Here's how the part is built. I have some questions about the finished solid (model axes, mm). A direction names the side the tool comes from. Coordinates: 2 decimals unless noted, no trailing zeros. Order: outer loops, then holes, each group sorted by start corner. A loop starts at its lowest first (then second) coordinate and runs counter-clockwise, first axis right, second up. Notation, with made-up numbers: (-4.5, 35.5) -> (7.5, 35.5) arc R21 cw to (7.5, 50.5) -> close; hole circle Ø10 at (39.5, 89). An arc over 180 degrees is marked (long way). One line per item, written item: value. Start each with the question number.
```python
from build123d import *

# Parameters (mm, degrees)
EXTRUDE_BASE_DEPTH              = 2
SKETCH2_W                       = 57
SKETCH2_H                       = 68.2942
EXTRUDE_WALLS_DEPTH             = 25
SKETCH3_W                       = 8.390953786
SKETCH3_H                       = 13
CUT_USB_HOLE_DEPTH              = 75.121635616
SKETCH4_R                       = 1.375
CUT_CONNECTING_THRU_HOLES_DEPTH = 75.121635616
SKETCH5_R                       = 2.25
SKETCH5_R_2                     = 1.375
CUT_EXTRUDE3_DEPTH              = 0.5
SKETCH6_R                       = 1.125
CUT_CABLE_COVER_BOTTOM_DEPTH    = 75.121635616
SKETCH7_R                       = 1.125
CUT_CABLE_COVER_SIDE_DEPTH      = 2
SKETCH8_W                       = 3.5
SKETCH8_H                       = 10
EXTRUDE_HINGE_DEPTH             = 4
SKETCH9_R                       = 1.125
CUT_HINGE_HOLE_DEPTH            = 85.478484791
FILLET_HINGE_R                  = 1.75
SKETCH10_W                      = 40
SKETCH10_H                      = 5
CUT_NOTCH_DEPTH                 = 1.5
SKETCH11_W                      = 10
SKETCH11_H                      = 5
CUT_SIDE_NOTCH_DEPTH            = 1.5
FILLET_NOTCH_R                  = 1.5


with BuildPart() as part:
    # Sketch1 → Extrude Base (new body)
    with BuildSketch(Plane.XZ.offset(-16.914945084)):
        with BuildLine():
            Line((56.857940404, 38.199863775), (56.857940404, -32.594336225))
            ThreePointArc((56.857940404, -32.594336225), (56.198930662, -34.185326483), (54.607940404, -34.844336225))
            Line((54.607940404, -34.844336225), (-4.892059596, -34.844336225))
            ThreePointArc((-4.892059596, -34.844336225), (-6.483049854, -34.185326483), (-7.142059596, -32.594336225))
            Line((-7.142059596, -32.594336225), (-7.142059596, 38.199863775))
            ThreePointArc((-7.142059596, 38.199863775), (-6.483049854, 39.790854032), (-4.892059596, 40.449863775))
            Line((-4.892059596, 40.449863775), (54.607940404, 40.449863775))
            ThreePointArc((54.607940404, 40.449863775), (56.198930662, 39.790854032), (56.857940404, 38.199863775))
        make_face()
    extrude(amount=EXTRUDE_BASE_DEPTH)

    # Sketch2 → Extrude Walls (add)
    with BuildSketch(Plane.XZ.offset(-14.914945084)):
        with BuildLine():
            Line((56.857940404, -32.594336225), (56.857940404, 38.199863775))
            ThreePointArc((56.857940404, 38.199863775), (56.198930662, 39.790854032), (54.607940404, 40.449863775))
            Line((54.607940404, 40.449863775), (-4.892059596, 40.449863775))
            ThreePointArc((-4.892059596, 40.449863775), (-6.483049854, 39.790854032), (-7.142059596, 38.199863775))
            Line((-7.142059596, 38.199863775), (-7.142059596, -32.594336225))
            ThreePointArc((-7.142059596, -32.594336225), (-6.483049854, -34.185326483), (-4.892059596, -34.844336225))
            Line((-4.892059596, -34.844336225), (54.607940404, -34.844336225))
            ThreePointArc((54.607940404, -34.844336225), (56.198930662, -34.185326483), (56.857940404, -32.594336225))
        make_face()
        with Locations((24.857940404, 2.802763775)):
            Rectangle(SKETCH2_W, SKETCH2_H, mode=Mode.SUBTRACT)
    extrude(amount=EXTRUDE_WALLS_DEPTH)

    # Sketch3 → Cut USB Hole (cut, through all)
    with BuildSketch(Plane.XZ.offset(-14.914945084)):
        with Locations((0.553417297, 27.849863775)):
            Rectangle(SKETCH3_W, SKETCH3_H)
    extrude(amount=-CUT_USB_HOLE_DEPTH, mode=Mode.SUBTRACT)

    # Sketch4 → Cut Connecting Thru Holes (cut, through all)
    with BuildSketch(Plane.XZ.offset(-14.914945084)):
        with Locations((50.982940404, 34.574863775)):
            Circle(SKETCH4_R)
        with Locations((50.982940404, -28.969336225)):
            Circle(SKETCH4_R)
        with Locations((-1.267059596, -28.969336225)):
            Circle(SKETCH4_R)
        with Locations((50.982940404, 2.802763775)):
            Circle(SKETCH4_R)
        with Locations((7.12389419, 21.124863775)):
            Circle(SKETCH4_R)
    extrude(amount=-CUT_CONNECTING_THRU_HOLES_DEPTH, mode=Mode.SUBTRACT)

    # Sketch5 → Cut-Extrude3 (cut)
    # profile 1 of 5: a face of its own
    with BuildSketch(Plane.XZ.offset(-14.914945084)):
        with Locations((7.12389419, 21.124863775)):
            Circle(SKETCH5_R)
        with Locations((7.12389419, 21.124863775)):
            Circle(SKETCH5_R_2, mode=Mode.SUBTRACT)
    # profile 2 of 5: a face of its own
    with BuildSketch(Plane.XZ.offset(-14.914945084)):
        with Locations((50.982940404, 34.574863775)):
            Circle(SKETCH5_R)
    # profile 3 of 5: a face of its own
    with BuildSketch(Plane.XZ.offset(-14.914945084)):
        with Locations((50.982940404, 2.802763775)):
            Circle(SKETCH5_R)
    # profile 4 of 5: a face of its own
    with BuildSketch(Plane.XZ.offset(-14.914945084)):
        with Locations((50.982940404, -28.969336225)):
            Circle(SKETCH5_R)
    # profile 5 of 5: a face of its own
    with BuildSketch(Plane.XZ.offset(-14.914945084)):
        with Locations((-1.267059596, -28.969336225)):
            Circle(SKETCH5_R)
    extrude(amount=-CUT_EXTRUDE3_DEPTH, mode=Mode.SUBTRACT)

    # Sketch6 → Cut Cable Cover Bottom (cut, through all)
    with BuildSketch(Plane.XZ.offset(-14.914945084)):
        with Locations((7.49889419, 34.199863775)):
            Circle(SKETCH6_R)
        with Locations((7.49889419, -8.594336225)):
            Circle(SKETCH6_R)
    extrude(amount=-CUT_CABLE_COVER_BOTTOM_DEPTH, mode=Mode.SUBTRACT)

    # Sketch7 → Cut Cable Cover Side (cut)
    with BuildSketch(Plane(origin=(-3.642059596, 0, 0), x_dir=(0, 0, -1), z_dir=(1, 0, 0))):
        with Locations(Location((8.594336225, 7.164945084, 0), (0, 0, 90))):
            Circle(SKETCH7_R)
        with Locations(Location((-34.199863775, 7.164945084, 0), (0, 0, 90))):
            Circle(SKETCH7_R)
    extrude(amount=-CUT_CABLE_COVER_SIDE_DEPTH, mode=Mode.SUBTRACT)

    # Sketch8 → Extrude Hinge (add)
    with BuildSketch(Plane.XZ.offset(10.085054916)):
        with Locations((55.107940404, -14.697236225)):
            Rectangle(SKETCH8_W, SKETCH8_H)
        with Locations((55.107940404, 20.302763775)):
            Rectangle(SKETCH8_W, SKETCH8_H)
    extrude(amount=EXTRUDE_HINGE_DEPTH)

    # Sketch9 → Cut Hinge Hole (cut, through all)
    with BuildSketch(Plane(origin=(0, 0, -19.697236225), x_dir=(-1, 0, 0), z_dir=(0, 0, -1))):
        with Locations((-55.107940404, -12.335054916)):
            Circle(SKETCH9_R)
    extrude(amount=-CUT_HINGE_HOLE_DEPTH, mode=Mode.SUBTRACT)

    # Fillet Hinge
    fillet_hinge_edges = [part.edges().sort_by_distance(p)[0] for p in [
        (56.857940404, -14.085054916, 20.302763775),
        (53.357940404, -14.085054916, 20.302763775),
        (56.857940404, -14.085054916, -14.697236225),
        (53.357940404, -14.085054916, -14.697236225),
    ]]
    fillet(fillet_hinge_edges, radius=FILLET_HINGE_R - 0.0001)  # a hair under: the kernel refuses the full size

    # Sketch10 → Cut Notch (cut)
    with BuildSketch(Plane(origin=(-3.642059596, 0, 0), x_dir=(0, 0, -1), z_dir=(1, 0, 0))):
        with Locations((-2.802763775, -2.585054916)):
            Rectangle(SKETCH10_W, SKETCH10_H)
    extrude(amount=-CUT_NOTCH_DEPTH, mode=Mode.SUBTRACT)

    # Sketch11 → Cut Side Notch (cut)
    with BuildSketch(Plane.XY.offset(-31.344336225)):
        with Locations((11.357940404, -2.585054916)):
            Rectangle(SKETCH11_W, SKETCH11_H)
    cut_side_notch = extrude(amount=-CUT_SIDE_NOTCH_DEPTH, mode=Mode.SUBTRACT)

    # Mirror Side Notch: Cut Side Notch across plane
    add(cut_side_notch.mirror(Plane(origin=(0, 0, 2.802763775), x_dir=(1, 0, 0), z_dir=(0, 0, -1))), mode=Mode.SUBTRACT)

    # Fillet Notch
    fillet_notch_edges = [part.edges().sort_by_distance(p)[0] for p in [
        (-5.142059596, -5.085054916, 2.802763775),
        (-5.142059596, -0.085054916, 2.802763775),
        (11.357940404, -5.085054916, -32.844336225),
        (11.357940404, -0.085054916, -32.844336225),
        (11.357940404, -5.085054916, 38.449863775),
        (11.357940404, -0.085054916, 38.449863775),
    ]]
    fillet(fillet_notch_edges, radius=FILLET_NOTCH_R - 0.0001)  # a hair under: the kernel refuses the full size


solid = part.part
```
Q1. For faces 1 (the face through (0, 16, 34.35)), 2 (the face through (11, -3, -32.844)), 3 (the face through (52.5, 15.415, -29.4)), 4 (the face through (55, -11, 25.303)), which set-ups out of +Z, -Z, +X, -X, +Y, -Y let a thin tool reach every point of the face, with its end or its side?
Q2. I need wall thicknesses on line 1 (X direction, y = 2.5, z = -27); line 2 (Z direction, x = 45, y = 6.5); line 3 (Z direction, x = -2.5, y = 15.5). Which ranges of each line are inside material? Lowest first, please.
Q3. Imagine slicing it at A-A (y = 9.5). Write out the boundary of the cut face in (x, z).
Q4. If we mould it in two halves opening along X, with no side actions, what happens to faces 5 (the face through (25, 16.915, 3)), 6 (the face through (-6.5, 3.6, -34.17)), 7 (the face through (56.232, -12.286, 20.233))? For each: +X half, -X half, draft (parallel to the pull), parting line (faces both ways), or undercut.
Q5. Imagine slicing it at B-B (x = 32). Write out the boundary of the cut face in (y, z), plus the area to 3 significant figures.
Q6. Imagine slicing it at C-C (z = -21). Write out the boundary of the cut face in (x, y).
Q7. For P1, Ø2.5, axis at x = 55.11, y = -12.34, coming from the -Z side; P2, Ø1.5, axis at x = 8, z = -4, coming from the -Y side; P3, Ø5, axis at x = 50.98, z = 34.57, coming from the +Y side, each with a flat end and sliding along its axis, tell me the tip position at first contact or that it passes through.
Completed:
1. face 1: +Y, -Y
1. face 2: none
1. face 3: -Y
1. face 4: +Z, +X, -X, -Y
2. line 1: x = -7.14 to -3.64, 53.36 to 56.86
2. line 2: z = -34.84 to -31.34, 36.95 to 40.45
2. line 3: z = -34.84 to -29.58, -28.36 to 21.35, 34.35 to 40.45
3. outline: (-7.14, -32.59) arc R2.25 ccw to (-4.89, -34.84) -> (54.61, -34.84) arc R2.25 ccw to (56.86, -32.59) -> (56.86, 38.2) arc R2.25 ccw to (54.61, 40.45) -> (-4.89, 40.45) arc R2.25 ccw to (-7.14, 38.2) -> close; hole (-3.64, -31.34) -> (53.36, -31.34) -> (53.36, 36.95) -> (-3.64, 36.95) -> close
4. face 5: draft
4. face 6: -X half
4. face 7: undercut
5. outline: (-10.09, -34.84) -> (16.91, -34.84) -> (16.91, 40.45) -> (-10.09, 40.45) -> (-10.09, 36.95) -> (14.91, 36.95) -> (14.91, -31.34) -> (-10.09, -31.34) -> close
5. area: 326 mm2
6. outline: (-7.14, -10.09) -> (-3.64, -10.09) -> (-3.64, 14.91) -> (53.36, 14.91) -> (53.36, -10.09) -> (56.86, -10.09) -> (56.86, 16.91) -> (-7.14, 16.91) -> close
7. P1: stops at z = -19.7
7. P2: stops at y = 14.91
7. P3: stops at y = 16.91
